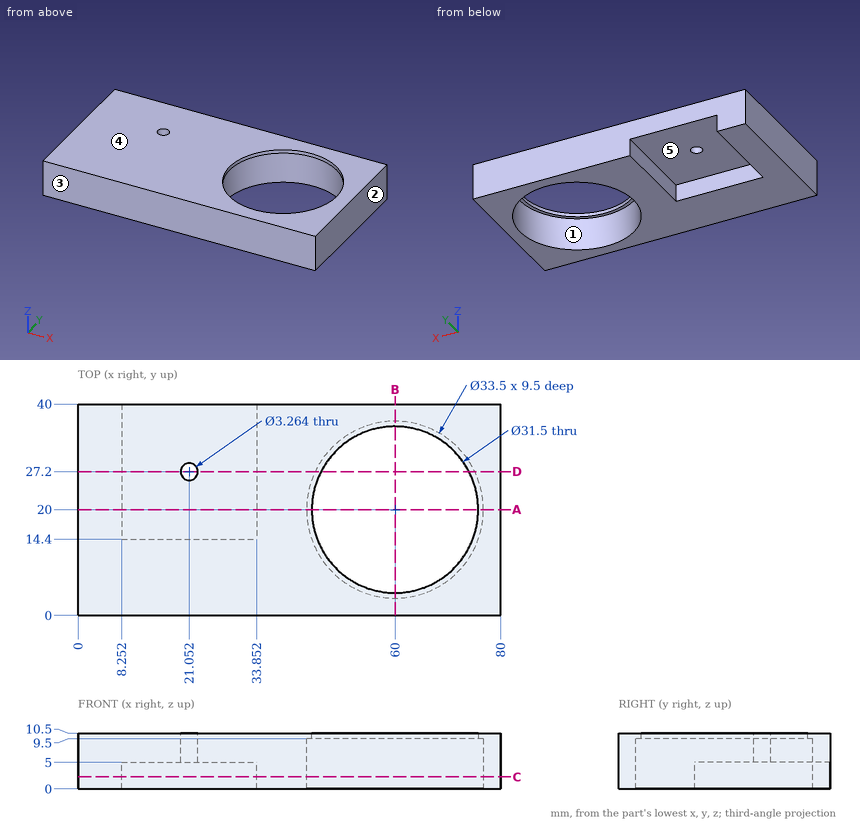
Check sheet for the drawn part. Datum: minimum x, y, z corner. Units: mm. A direction names the side the tool comes from. Round coordinates to 2 decimals unless told otherwise and drop trailing zeros. Order: outer loops, then holes, each group sorted by start corner. A loop starts at its lowest first (then second) coordinate and runs counter-clockwise, first axis right, second up. Notation, with made-up numbers: M 22.25,55.5 L 54.25,55.5 A17 cw 54.25,76.5 Z; hole C -34.5,-36 d8. An arc over 180 degrees is marked long. Answer in a Markdown table with one row per item.
(1) Set-up check for the marked faces 4 and 5: record each of +Z, -Z, +X, -X, +Y, -Y from which the full face is reachable in a straight line by a thin tool's end or side.
Findings:
| item | result |
|---|---|
| face 4 | +Z, +X, -X, +Y, -Y |
| face 5 | -Z, +Y |
(2) Section check C-C on z = 2.25. Record the boundary of the cut face in (x, y), plus the area to 3 significant figures.
Findings:
| item | result |
|---|---|
| outline | M 0,0 L 80,0 L 80,40 L 33.85,40 L 33.85,14.4 L 8.25,14.4 L 8.25,40 L 0,40 Z; hole C 60,20 d33.5 |
| area | 1,660 mm^2 |
(3) Material ranges on line 1 along X through (y, z) = (20.5, 4.5); line 2 along X through (y, z) = (24.5, 2.5); line 3 along Y through (x, z) = (60, 3), recorded low to high. Write a range as from..to.
Findings:
| item | result |
|---|---|
| line 1 | x = 0..8.25, 33.85..43.26, 76.74..80 |
| line 2 | x = 0..8.25, 33.85..43.87, 76.13..80 |
| line 3 | y = 0..3.25, 36.75..40 |
(4) Section check D-D on y = 27.2. Record the boundary of the cut face in (x, z).
Findings:
| item | result |
|---|---|
| outline | M 0,0 L 8.25,0 L 8.25,5 L 19.42,5 L 19.42,10.5 L 0,10.5 Z; M 22.68,5 L 33.85,5 L 33.85,0 L 44.88,0 L 44.88,9.5 L 45.99,9.5 L 45.99,10.5 L 22.68,10.5 Z; M 74.01,9.5 L 75.12,9.5 L 75.12,0 L 80,0 L 80,10.5 L 74.01,10.5 Z |
(5) Gauge pin test, flat ends, axial feed: pin 1 (2 mm diameter, centred on x = 13.5, y = 15.5, fed in from -Z); pin 2 (1.5 mm diameter, centred on x = 25.5, z = 1.5, fed in from +Y). Record the tip position at first contact, or that the pin passes through.
Findings:
| item | result |
|---|---|
| pin 1 | stops at z = 5 |
| pin 2 | stops at y = 14.4 |
(6) Section check A-A on y = 20. Record the boundary of the cut face in (x, z), plus the area to 3 significant figures.
Findings:
| item | result |
|---|---|
| outline | M 0,0 L 8.25,0 L 8.25,5 L 33.85,5 L 33.85,0 L 43.25,0 L 43.25,9.5 L 44.25,9.5 L 44.25,10.5 L 0,10.5 Z; M 75.75,9.5 L 76.75,9.5 L 76.75,0 L 80,0 L 80,10.5 L 75.75,10.5 Z |
| area | 362 mm^2 |
(7) Section check B-B on x = 60. Record the boundary of the cut face in (y, z).
Findings:
| item | result |
|---|---|
| outline | M 0,0 L 3.25,0 L 3.25,9.5 L 4.25,9.5 L 4.25,10.5 L 0,10.5 Z; M 35.75,9.5 L 36.75,9.5 L 36.75,0 L 40,0 L 40,10.5 L 35.75,10.5 Z |
(8) Draft check along X on the marked faces 1, 2 and 3. Enter one of: +X half, -X half, draft (parallel to the pull), parting line (faces both ways), or undercut.
Findings:
| item | result |
|---|---|
| face 1 | undercut |
| face 2 | +X half |
| face 3 | draft |
